from build123d import *

# Parameters (mm, degrees)
SKETCH_W        = 9.5
SKETCH_H        = 6.05
PAD_DEPTH       = 14.5
FILLET_R        = 3
SKETCH001_R     = 1
POCKET_DEPTH    = 0.5
SKETCH003_W     = 2.8
SKETCH003_H     = 2.8
POCKET001_DEPTH = 14


with BuildPart() as part:
    # Sketch → Pad (new body)
    with BuildSketch(Plane.XY):
        Rectangle(SKETCH_W, SKETCH_H)
    extrude(amount=PAD_DEPTH)

    # Fillet
    fillet_edges = [part.edges().sort_by_distance(p)[0] for p in [
        (-4.75, -3.025, 7.25),
        (4.75, -3.025, 7.25),
        (4.75, 3.025, 7.25),
        (-4.75, 3.025, 7.25),
    ]]
    fillet(fillet_edges, radius=FILLET_R)

    # Sketch001 (on Face2 of Fillet) → Pocket (cut)
    with BuildSketch(Plane(origin=(0, 0, 0), x_dir=(1, 0, 0), z_dir=(0, 0, -1))):
        with Locations((1.8, 0)):
            Circle(SKETCH001_R)
        with Locations((-1.8, 0)):
            Circle(SKETCH001_R)
    extrude(amount=-POCKET_DEPTH, mode=Mode.SUBTRACT)

    # Sketch003 (on Face14 of Pocket) → Pocket001 (cut)
    with BuildSketch(Plane(origin=(0, 0, 0.5), x_dir=(1, 0, 0), z_dir=(0, 0, -1))):
        with Locations((1.8, 0)):
            Rectangle(SKETCH003_W, SKETCH003_H)
        with Locations((-1.8, 0)):
            Rectangle(SKETCH003_W, SKETCH003_H)
    extrude(amount=-POCKET001_DEPTH, mode=Mode.SUBTRACT)


solid = part.part
Verification items for the finished model (mm, model axes). A direction names the side the tool comes from. Give positions to 0.01 mm unless a question says otherwise; leave off trailing zeros. Write each loop counter-clockwise with the first axis right and the second up, starting at its lowest first coordinate (ties: lowest second). Pieces come first, ordered by that corner, then holes.
(1) Material ranges on line 1 (X direction, y = 0, z = 0.35); line 2 (X direction, y = 0, z = 8.5); line 3 (Y direction, x = -1.8, z = 0.35), recorded low to high.
(2) Cross-section at B-B (x = -2.25). Enter the section's corners in (y, z).
(3) Cross-section at A-A (z = 10.25). Enter the section's corners in (x, y) (3 decimals), plus the area to 3 significant figures.
(4) Cross-section at C-C (y = -2.25). Enter the section's corners in (x, z).
(5) Mould release check, pull along Y, two halves, no side actions. Record for faces 1 (the face through (0.4, 0, 7)), 2 (the face through (-0.4, 0, 7)), 3 (the face through (0, 0, 0)), 4 (the face through (-3.895, 2.123, 7.352)): +Y half, -Y half, draft (parallel to the pull), parting line (faces both ways), or undercut.
(6) Access from +Z, -Z, +X, -X, +Y, -Y to the whole of each face (thin tool, end or side, straight path). Record for faces 5 (the face through (0, 0, 14.5)), 6 (the face through (2, 1.4, 7)).
(7) Gauge pin test, flat ends, axial feed: pin 1 (1.5 mm diameter, centred on y = -2, z = 4.5, fed in from -X); pin 2 (2 mm diameter, centred on x = -2, y = 0, fed in from +Z); pin 3 (1 mm diameter, centred on y = -2.5, z = 3, fed in from -X). Record the tip position at first contact, or that the pin passes through.
Worked out:
1. line 1: x = -4.75 to -2.8, -0.8 to 0.8, 2.8 to 4.75
1. line 2: x = -4.75 to -3.2, -0.4 to 0.4, 3.2 to 4.75
1. line 3: y = -3.02 to -1, 1 to 3.02
2. outline: (-2.98, 0) - (-0.89, 0) - (-0.89, 0.5) - (-1.4, 0.5) - (-1.4, 14.5) - (-2.98, 14.5) - close; (0.89, 0) - (2.98, 0) - (2.98, 14.5) - (1.4, 14.5) - (1.4, 0.5) - (0.89, 0.5) - close
3. outline: (-4.75, -0.025) arc R3 ccw to (-1.75, -3.025) - (1.75, -3.025) arc R3 ccw to (4.75, -0.025) - (4.75, 0.025) arc R3 ccw to (1.75, 3.025) - (-1.75, 3.025) arc R3 ccw to (-4.75, 0.025) - close; hole (-3.2, -1.4) - (-0.4, -1.4) - (-0.4, 1.4) - (-3.2, 1.4) - close; hole (0.4, -1.4) - (3.2, -1.4) - (3.2, 1.4) - (0.4, 1.4) - close
3. area: 34.1 mm2
4. outline: (-3.76, 0) - (3.76, 0) - (3.76, 14.5) - (-3.76, 14.5) - close
5. face 1: undercut
5. face 2: undercut
5. face 3: draft
5. face 4: +Y half
6. face 5: +Z, +X, -X, +Y, -Y
6. face 6: +Z
7. pin 1: stops at x = -4.49
7. pin 2: stops at z = 0.5
7. pin 3: stops at x = -4.01
